from build123d import *

# Parameters (mm, degrees)
F0_W        = 14.224
F0_H        = 12.065
F0_W_2      = 9.144
F0_H_2      = 6.985
F1_DEPTH    = 25.4
F3_DEPTH    = 8.89
F5_DEPTH    = 25.4
F6_T1_DEPTH = 37.465


# Not quite as in the source:
# - a fillet or chamfer that OpenCascade refuses, or shapes differently, is made with other operations: its cross-section is extruded or revolved along the edge and cut away or added


with BuildPart() as f1:
    # F0 (on Top) → F1 (new body)
    with BuildSketch(Plane.XY):
        Rectangle(F0_W, F0_H)
        Rectangle(F0_W_2, F0_H_2, mode=Mode.SUBTRACT)
    extrude(amount=F1_DEPTH)

    # F2 (on face) → F3 (join)
    with BuildSketch(Plane(origin=(0, -3.4925, 0), x_dir=(-1, 0, 0), z_dir=(0, 1, 0))):
        with BuildLine():
            Line((3.801523905, 13.97), (-3.801523905, 13.97))
            ThreePointArc((-3.801523905, 13.97), (-4.3751429287, 12.7571429287), (-4.572, 11.43))
            Line((-4.572, 11.43), (4.572, 11.43))
            ThreePointArc((4.572, 11.43), (4.3751429287, 12.7571429287), (3.801523905, 13.97))
        make_face()
        with BuildLine():
            Line((-3.801523905, 13.97), (-4.572, 13.97))
            Line((-4.572, 13.97), (-4.572, 11.43))
            ThreePointArc((-4.572, 11.43), (-4.3751429287, 12.7571429287), (-3.801523905, 13.97))
        make_face()
        with BuildLine():
            Line((4.572, 13.97), (3.801523905, 13.97))
            ThreePointArc((3.801523905, 13.97), (4.3751429287, 12.7571429287), (4.572, 11.43))
            Line((4.572, 11.43), (4.572, 13.97))
        make_face()
        with BuildLine():
            Line((4.572, 11.43), (-4.572, 11.43))
            ThreePointArc((-4.572, 11.43), (0, 6.858), (4.572, 11.43))
        make_face()
    extrude(amount=F3_DEPTH)

    # F4 (on face) → F5 (cut)
    with BuildSketch(Plane(origin=(0, 6.0325, 0), x_dir=(-1, 0, 0), z_dir=(0, 1, 0))):
        with BuildLine():
            ThreePointArc((-1.5709032434, 25.4), (-1.784854865, 19.424145135), (3.429, 22.352))
            ThreePointArc((3.429, 22.352), (2.927854865, 24.136854865), (1.5709032434, 25.4))
            Line((1.5709032434, 25.4), (-1.5709032434, 25.4))
        make_face()
    extrude(amount=-F5_DEPTH, mode=Mode.SUBTRACT)

    # F6: fillet of radius 5.08 on 2 edges, made by hand

    # F6_s2 → F6_t1 (cut)
    with BuildSketch(Plane.XZ.offset(-18.7325)):
        with BuildLine():
            ThreePointArc((7.112, 20.32), (5.6241024484, 23.9121024484), (2.032, 25.4))
            Line((2.032, 25.4), (7.112, 25.4))
            Line((7.112, 25.4), (7.112, 20.32))
        make_face()
        with BuildLine():
            ThreePointArc((-2.032, 25.4), (-5.6241024484, 23.9121024484), (-7.112, 20.32))
            Line((-7.112, 20.32), (-7.112, 25.4))
            Line((-7.112, 25.4), (-2.032, 25.4))
        make_face()
    extrude(amount=F6_T1_DEPTH, mode=Mode.SUBTRACT)


solid = f1.part
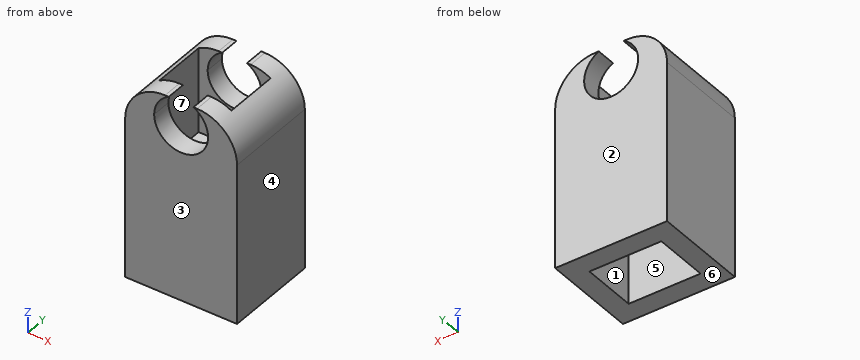
Input: part model. Units: mm. Frame: model coordinates. Face numbers are marked on the shaded views. A direction names the side the tool comes from. Coordinates: 2 decimals unless noted, no trailing zeros. Order: outer loops, then holes, each group sorted by start corner. A loop starts at its lowest first (then second) coordinate and runs counter-clockwise, first axis right, second up. Notation, with made-up numbers: M -7,-19 L 30,-19 A20 cw 30,5 Z; hole C -15.5,27.5 d8. An arc over 180 degrees is marked long. One line per question, with ' | ' between items.
Item 1: Section D-D (z = 23.75). Output: boundary loops of the cut face in (x, y), then the cut area to 3 significant figures.
Geometry results:
outline: M -5.78,-6.03 L -3.13,-6.03 L -3.13,-3.49 L -4.57,-3.49 L -4.57,3.49 L -3.13,3.49 L -3.13,6.03 L -5.78,6.03 Z; M 3.13,-6.03 L 5.78,-6.03 L 5.78,6.03 L 3.13,6.03 L 3.13,3.49 L 4.57,3.49 L 4.57,-3.49 L 3.13,-3.49 Z | area: 43.8 mm^2
Item 2: Section B-B (y = 0.75). Output: boundary loops of the cut face in (x, z).
Geometry results:
outline: M -7.11,0 L -4.57,0 L -4.57,11.43 A4.57 ccw 4.57,11.43 L 4.57,0 L 7.11,0 L 7.11,20.32 A5.08 ccw 4.57,24.72 L 4.57,13.97 L -4.57,13.97 L -4.57,24.72 A5.08 ccw -7.11,20.32 Z
Item 3: Draft query along Y for the marked faces 1, 2, 3 and 4. Return one class per face: released by +Y, released by -Y, zero draft, split by the parting line, or undercut.
Geometry results:
face 1: undercut | face 2: released by +Y | face 3: released by -Y | face 4: zero draft
Item 4: Ray query, line 1 along Y through (x, z) = (-3.5, 6.5); line 2 along X through (y, z) = (-2.5, 8.25); line 3 along X through (y, z) = (1.75, 15.75). Return the intervals inside material, ascending.
Geometry results:
line 1: y = -6.03 to -3.49, 3.49 to 6.03 | line 2: x = -7.11 to -4.57, -3.28 to 3.28, 4.57 to 7.11 | line 3: x = -7.11 to -4.57, 4.57 to 7.11
Item 5: Pin query (flat end, axial travel): pin 1 (3.5 mm diameter, centred on x = 0.5, y = 1.5, fed in from +Z); pin 2 (3 mm diameter, centred on x = 4, y = 1.5, fed in from +Z). Return the tip coordinate at first contact, or that it passes through.
Geometry results:
pin 1: stops at z = 13.97 | pin 2: stops at z = 24.72
Item 6: Reachability of the marked faces 5, 6 and 7 from +Z, -Z, +X, -X, +Y, -Y: full face, straight path, thin tool, end or side. Return the list, or none.
Geometry results:
face 5: -Z | face 6: -Z, +X, -X, +Y, -Y | face 7: +Z
Item 7: Section C-C (x = 0). Output: boundary loops of the cut face in (y, z).
Geometry results:
outline: M -6.03,0 L -3.49,0 L -3.49,6.86 L 3.49,6.86 L 3.49,0 L 6.03,0 L 6.03,18.92 L 3.49,18.92 L 3.49,13.97 L -3.49,13.97 L -3.49,18.92 L -6.03,18.92 Z
Item 8: Section A-A (z = 5.25). Output: boundary loops of the cut face in (x, y).
Geometry results:
outline: M -7.11,-6.03 L 7.11,-6.03 L 7.11,6.03 L -7.11,6.03 Z; hole M -4.57,-3.49 L 4.57,-3.49 L 4.57,3.49 L -4.57,3.49 Z
